Autodesk Inventor part; units mm, degrees
ref_plane "YZ Plane" through (0, 0, 0) normal (1, 0, 0) x (0, 1, 0)
ref_plane "XZ Plane" through (0, 0, 0) normal (0, 1, 0) x (-1, 0, 0)
ref_plane "XY Plane" through (0, 0, 0) normal (0, 0, 1) x (1, 0, 0)
sketch "Sketch1" plane through (0, 0, 0) normal (0, 0, 1) x (1, 0, 0)
  circle A0 centre (0, 0) radius 6.35
  circle A1 centre (0, 0) radius 8.7313
  circle A2 centre (0, 0) radius 7.9375
  dimension "d0" = 12.7
  dimension "d3" = 17.4625
  dimension "d4" = 0.7937
extrude "Extrusion1" add sketch "Sketch1" along normal blind 1.5875 contours A0 | A1 | A2
sketch "Sketch2" plane through (0, 0, 1.5875) normal (0, 0, 1) x (1, 0, 0)
  circle A0 centre (0, 0) radius 6.35
  circle A1 centre (0, 0) radius 8.7313
  circle A2 centre (0, 0) radius 7.9375
  dimension "d7" = 12.7
  dimension "d8" = 17.4625
  dimension "d9" = 0.7937
extrude "Extrusion2" add sketch "Sketch2" along normal blind 1.5875 contours A2
sketch "Sketch3" plane through (0, 0, 1.5875) normal (0, 0, 1) x (1, 0, 0)
  circle A0 centre (0, 0) radius 6.35
  circle A1 centre (0, 0) radius 6.35
extrude "Extrusion3" cut sketch "Sketch3" against normal blind 3.175
sketch "Sketch4" plane through (0, 0, 3.175) normal (0, 0, 1) x (1, 0, 0)
  circle A0 centre (0, 0) radius 7.9375
  circle A1 centre (0, 0) radius 7.9375
  circle A2 centre (0, 0) radius 7.1438
  dimension "d14" = 0.7937
extrude "Extrusion4" add sketch "Sketch4" along normal blind 1.5875
properties part number "Needle Bearing Stopper"
Model file for the job. Use its own axes, mm. A direction names the side the tool comes from. Coordinates: 2 decimals unless noted, no trailing zeros. Order: outer loops, then holes, each group sorted by start corner. A loop starts at its lowest first (then second) coordinate and runs counter-clockwise, first axis right, second up. Notation, with made-up numbers: M -22,66 L 2,66 A27 cw 2,89 Z; hole C 73,24 d2. An arc over 180 degrees is marked long. Answer as CSV lines item,"result".
(1) Pull direction X, two halves, no side cores. Call faces 1 (the flat face through (-6, -3, 3.175)), 2 (the flat face through (2, -8, 1.588)), 3 (the cylindrical face through (-1.38, 6.2, 1.57)), 4 (the cylindrical face through (-1.72, 7.75, 3.15)): +X half, -X half, draft (parallel to the pull), parting line (faces both ways), or undercut.
Geometry says:
face 1,"undercut"
face 2,"draft"
face 3,"undercut"
face 4,"parting line"
(2) 3-axis set-ups, long thin cutter, end or side, ignore diameter. For faces 5 (the cylindrical face through (-5.669, 4.347, 3.958)), 6 (the flat face through (-6, -3, 0)): which of +Z, -Z, +X, -X, +Y, -Y reach the whole face in a straight line?
Geometry says:
face 5,"+Z"
face 6,"-Z, +X, -X, +Y, -Y"
(3) Wall check: line 1 along Y through (x, z) = (0, 2.1); line 2 along Y through (x, z) = (0, 4.35); line 3 along X through (y, z) = (5, 1.9). Give the ranges that are in metal, low to high.
Geometry says:
line 1,"y = -7.94 to -6.35, 6.35 to 7.94"
line 2,"y = -7.94 to -7.14, 7.14 to 7.94"
line 3,"x = -6.16 to -3.91, 3.91 to 6.16"
(4) Flat gauge pins, fed straight in: pin 1 (1.5 mm diameter, centred on x = -5.5, z = 1, fed in from +Y); pin 2 (5 mm diameter, centred on x = 0.5, y = 2.5, fed in from +Z); pin 3 (5 mm diameter, centred on x = -2.5, y = 3, fed in from +Z) (3 decimals). Where does each tip first touch, or does it go through?
Geometry says:
pin 1,"stops at y = 7.33"
pin 2,"passes through"
pin 3,"stops at z = 3.175"
(5) Band-saw the part on D-D, the plane x = 7.5. List the corners of the cut face in (y, z), then the cut area to 3 significant figures.
Geometry says:
outline,"M -4.47,0 L 4.47,0 L 4.47,1.59 L 2.6,1.59 L 2.6,4.76 L -2.6,4.76 L -2.6,1.59 L -4.47,1.59 Z"
area,"30.7 mm2"
